Can you work these out from the model? Positions are in its coordinate system, mm. A direction names the side the tool comes from. Round coordinates to 2 decimals unless told otherwise and drop trailing zeros. Loops run counter-clockwise (first coordinate to the right, second up) from the corner with the lowest first, then second, coordinate; pieces in that order, holes last.
(1) I want a section at A-A on x = 0. Write out the boundary of the cut face in (y, z).
(2) Will these pins go through, and if not, where does the flat tip stop? pin 1 Ø5 at (x, z) = (-128, 68) entering from +Y; pin 2 Ø1.5 at (x, z) = (348, 36.5) entering from +Y; pin 3 Ø6 at (x, z) = (131, 9) entering from -Y; pin 4 Ø8 at (y, z) = (-6.5, 56.5) entering from -X.
(3) Which directions (+Z, -Z, +X, -X, +Y, -Y) give clear straight access to the entire face, cutting with the end or side of a thin tool? Please do faces 4 (the face through (-128.982, -131.727, 37.325)), 5 (the face through (-88, 204, 50)), 6 (the face through (-2, -248, 52)).
(4) I want a section at D-D on x = -235. Write out the boundary of the cut face in (y, z).
(5) I want a section at C-C on z = 11. Write out the boundary of the cut face in (x, y).
(6) I want a section at B-B on y = 0. Write out the boundary of the cut face in (x, z).
(7) Thinking about a two-plate mould opening in Y: for faces 1 (the face through (-219, 53, 52)), 2 (the face through (-68.503, 195.605, 64.325)), 3 (the face through (345, 204, 50)), which applies, released by +Y, released by -Y, zero draft, split by the parting line, or undercut?
(8) If I drill on line 1 along Z through (x, y) = (-243, 333); line 2 along Z through (x, y) = (-80, 332); line 3 along Z through (x, y) = (-257.5, 26.5), over which ranges is the centre line in solid material (lowest first)?
from build123d import *

# Parameters (mm, degrees)
F0_R     = 450
F1_DEPTH = 25
F2_R     = 175
F3_DEPTH = 25
F4_R     = 150
F5_DEPTH = 2
F6_R     = 150
F7_DEPTH = 25


with BuildPart() as f1:
    # F0 (on Top) → F1 (new body)
    with BuildSketch(Plane.XY):
        Circle(F0_R)
    extrude(amount=F1_DEPTH)

    # F2 (on face) → F3 (join)
    with BuildSketch(Plane.XY.offset(25)):
        with Locations((0, -250)):
            Circle(F2_R)
        with Locations((-216.506351, 125)):
            Circle(F2_R)
        with Locations((216.506351, 125)):
            Circle(F2_R)
    extrude(amount=F3_DEPTH)

    # F4 (on face) → F5 (join)
    with BuildSketch(Plane.XY.offset(50)):
        with Locations((-216.506351, 125)):
            Circle(F4_R)
        with Locations((216.506351, 125)):
            Circle(F4_R)
        with Locations((0, -250)):
            Circle(F4_R)
    extrude(amount=F5_DEPTH)

    # F6 (on face) → F7 (join)
    with BuildSketch(Plane.XY.offset(52)):
        with BuildLine():
            ThreePointArc((-74.225818, 172.5), (-68.448795, 195.938411), (-66.506351, 220))
            ThreePointArc((-66.506351, 220), (-240.567939, 368.057556), (-358.786884, 172.5))
            ThreePointArc((-358.786884, 172.5), (-216.506351, 275), (-74.225818, 172.5))
        make_face()
        with BuildLine():
            ThreePointArc((-74.225818, 172.5), (-216.506351, 275), (-358.786884, 172.5))
            ThreePointArc((-358.786884, 172.5), (-216.506351, 70), (-74.225818, 172.5))
        make_face()
        with Locations((216.508, 220)):
            Circle(F6_R)
    extrude(amount=F7_DEPTH)


solid = f1.part
Filled sheet:
1. outline: (-450, 0) - (450, 0) - (450, 25) - (-75, 25) - (-75, 50) - (-100, 50) - (-100, 52) - (-400, 52) - (-400, 50) - (-425, 50) - (-425, 25) - (-450, 25) - close
2. pin 1: stops at y = 342.89
2. pin 2: stops at y = 241.32
2. pin 3: stops at y = -431.41
2. pin 4: passes through
3. face 4: +Z
3. face 5: none
3. face 6: +Z, +X, -X, -Y
4. outline: (-383.76, 0) - (383.76, 0) - (383.76, 25) - (299.02, 25) - (299.02, 50) - (273.86, 50) - (273.86, 52) - (368.86, 52) - (368.86, 77) - (71.14, 77) - (71.14, 52) - (-23.86, 52) - (-23.86, 50) - (-49.02, 50) - (-49.02, 25) - (-383.76, 25) - close
5. outline: circle Ø900 at (0, 0)
6. outline: (-450, 0) - (450, 0) - (450, 25) - (338.98, 25) - (338.98, 50) - (299.42, 50) - (299.42, 52) - (133.59, 52) - (133.59, 50) - (94.03, 50) - (94.03, 25) - (-94.03, 25) - (-94.03, 50) - (-133.59, 50) - (-133.59, 52) - (-299.42, 52) - (-299.42, 50) - (-338.98, 50) - (-338.98, 25) - (-450, 25) - close
7. face 1: zero draft
7. face 2: released by -Y
7. face 3: undercut
8. line 1: z = 0 to 25, 52 to 77
8. line 2: z = 0 to 25
8. line 3: z = 0 to 52
